Autodesk Inventor part; units mm, degrees
sketch "Эскиз1" plane through (0, 0, 0) normal (0, 0, 1) x (1, 0, 0)
  line L0 (-21, -9.25) -> (21, -9.25)
  line L1 (21, -9.25) -> (21, 9.25)
  line L2 (21, 9.25) -> (-21, 9.25)
  line L3 (-21, 9.25) -> (-21, -9.25)
  line L4 (-21, -9.25) -> (21, 9.25) construction
  line L5 (21, -9.25) -> (-21, 9.25) construction
  point P0 (0, 0)
  dimension "d0" = 42
  dimension "d1" = 18.5
extrude "Выдавливание1" add sketch "Эскиз1" along normal mid plane 2
sketch "Эскиз2" plane through (0, 0, 1) normal (0, 0, 1) x (1, 0, 0)
  circle A0 centre (-16.5, 0) radius 1.65
  circle A1 centre (16.5, 0) radius 1.65
  point P0 (0, 0)
extrude "Выдавливание2" cut sketch "Эскиз2" against normal up to next
properties part number "Фиксатор"
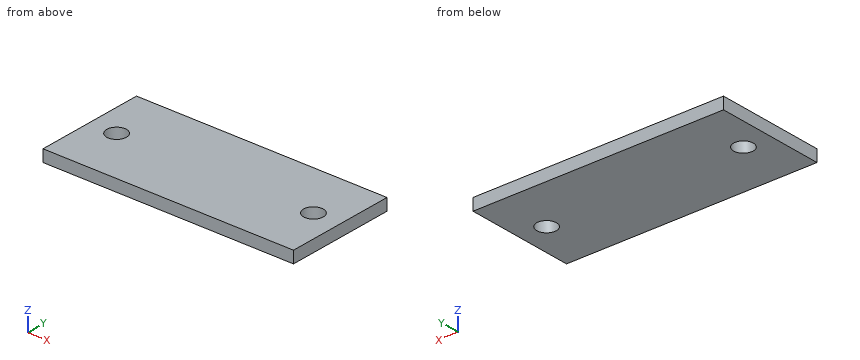
Design review of the part built by this model. Coordinates are the model's own, in mm. Give positions to 0.01 mm unless a question says otherwise; leave off trailing zeros. Write each loop counter-clockwise with the first axis right and the second up, starting at its lowest first coordinate (ties: lowest second). Pieces come first, ordered by that corner, then holes. Notation, with made-up numbers: M 60,-21 L 82,-21 A20 cw 82,10 Z; hole C -22.5,69 d3. An arc over 180 degrees is marked long. Return JSON: item names as keys, results as strings. Group by question number.
Item 1: Take a section at C-C (z = -0.5). Give the boundary of the cut face in (x, y), plus the area to 3 significant figures.
Item 2: Wall thickness on line 1 along Y through (x, z) = (16.5, -0.5); line 2 along X through (y, z) = (-1, 0.6); line 3 along Y through (x, z) = (-17.5, 0.55): over which ranges is each line inside the solid? List them lowest first.
Item 3: Clearance check with a flat-ended pin moving along its axis: pin 1 Ø3 at (x, y) = (-16.5, 0) entering from -Z. State where the tip first meets the part, or that it passes through.
Item 4: Take a section at B-B (x = 16.5). Give the boundary of the cut face in (y, z), plus the area to 3 significant figures.
Item 5: Take a section at A-A (y = 0). Give the boundary of the cut face in (x, z).
Return value:
{
 "1": {"outline": "M -21,-9.25 L 21,-9.25 L 21,9.25 L -21,9.25 Z; hole C -16.5,0 d3.3; hole C 16.5,0 d3.3", "area": "760 mm2"},
 "2": {"line 1": "y = -9.25 to -1.65, 1.65 to 9.25", "line 2": "x = -21 to -17.81, -15.19 to 15.19, 17.81 to 21", "line 3": "y = -9.25 to -1.31, 1.31 to 9.25"},
 "3": {"pin 1": "passes through"},
 "4": {"outline": "M -9.25,-1 L -1.65,-1 L -1.65,1 L -9.25,1 Z; M 1.65,-1 L 9.25,-1 L 9.25,1 L 1.65,1 Z", "area": "30.4 mm2"},
 "5": {"outline": "M -21,-1 L -18.15,-1 L -18.15,1 L -21,1 Z; M -14.85,-1 L 14.85,-1 L 14.85,1 L -14.85,1 Z; M 18.15,-1 L 21,-1 L 21,1 L 18.15,1 Z"}
}
